```python
from build123d import *

# Parameters (mm, degrees)
F0_R     = 6
F1_DEPTH = 5
F2_DEPTH = 3
F3_W     = 34
F3_H     = 50
F4_DEPTH = 2
F5_R     = 1.155008
F5_R_2   = 1.094696
F5_R_3   = 1.161259
F5_R_4   = 0.979267
F6_DEPTH = 3.001


with BuildPart() as f1:
    # F0 (on Top) → F1 (new body)
    with BuildSketch(Plane.XY):
        with BuildLine():
            ThreePointArc((83.212636, 86.809125), (44.989895, 73.04652), (6.710183, 86.64986))
            ThreePointArc((6.710183, 86.64986), (-5.47746, 95.123225), (3.790625, 83.528434))
            ThreePointArc((3.790625, 83.528434), (15.91287, 45.057288), (3.24039, 6.763865))
            ThreePointArc((3.24039, 6.763865), (-5.358143, -5.247885), (6.829769, 3.099073))
            ThreePointArc((6.829769, 3.099073), (45.077454, 16.173317), (83.585051, 3.88567))
            ThreePointArc((83.585051, 3.88567), (94.910037, -5.66935), (87.070277, 6.904109))
            ThreePointArc((87.070277, 6.904109), (75.1752, 45.066281), (86.359609, 83.442748))
            ThreePointArc((86.359609, 83.442748), (95.478836, 95.121753), (83.212636, 86.809125))
        make_face()
        Circle(F0_R, mode=Mode.SUBTRACT)
        with Locations((90, 0)):
            Circle(F0_R, mode=Mode.SUBTRACT)
        with BuildLine():
            ThreePointArc((85.006812, 84.403744), (71.302344, 45), (85.006812, 5.596256))
            ThreePointArc((85.006812, 5.596256), (84.696699, 5.303301), (84.403744, 4.993188))
            ThreePointArc((84.403744, 4.993188), (45, 18.697656), (5.596256, 4.993188))
            ThreePointArc((5.596256, 4.993188), (5.303301, 5.303301), (4.993188, 5.596256))
            ThreePointArc((4.993188, 5.596256), (18.697656, 45), (4.993188, 84.403744))
            ThreePointArc((4.993188, 84.403744), (5.303301, 84.696699), (5.596256, 85.006812))
            ThreePointArc((5.596256, 85.006812), (45, 71.302344), (84.403744, 85.006812))
            ThreePointArc((84.403744, 85.006812), (84.696699, 84.696699), (85.006812, 84.403744))
        make_face(mode=Mode.SUBTRACT)
        with Locations((0, 90)):
            Circle(F0_R, mode=Mode.SUBTRACT)
        with Locations((90, 90)):
            Circle(F0_R, mode=Mode.SUBTRACT)
    extrude(amount=F1_DEPTH)

    # F0 (on Top) → F2 (join)
    with BuildSketch(Plane.XY):
        with BuildLine():
            ThreePointArc((84.403744, 4.993188), (84.696699, 5.303301), (85.006812, 5.596256))
            ThreePointArc((85.006812, 5.596256), (71.302344, 45), (85.006812, 84.403744))
            ThreePointArc((85.006812, 84.403744), (84.696699, 84.696699), (84.403744, 85.006812))
            ThreePointArc((84.403744, 85.006812), (45, 71.302344), (5.596256, 85.006812))
            ThreePointArc((5.596256, 85.006812), (5.303301, 84.696699), (4.993188, 84.403744))
            ThreePointArc((4.993188, 84.403744), (18.697656, 45), (4.993188, 5.596256))
            ThreePointArc((4.993188, 5.596256), (5.303301, 5.303301), (5.596256, 4.993188))
            ThreePointArc((5.596256, 4.993188), (45, 18.697656), (84.403744, 4.993188))
        make_face()
    extrude(amount=F2_DEPTH)

    # F3 (on face) → F4 (cut)
    with BuildSketch(Plane.XY.offset(3)):
        with Locations((45, 45)):
            Rectangle(F3_W, F3_H)
    extrude(amount=-F4_DEPTH, mode=Mode.SUBTRACT)

    # F5 (on face) → F6 (cut, through all)
    with BuildSketch(Plane.XY.offset(3)):
        with Locations((59.727397, 21.745855)):
            Circle(F5_R)
        with Locations((29.705523, 68.703085)):
            Circle(F5_R_2)
        with Locations((29.668592, 21.745855)):
            Circle(F5_R_3)
        with Locations((59.817981, 68.572104)):
            Circle(F5_R_4)
    extrude(amount=-F6_DEPTH, mode=Mode.SUBTRACT)


solid = f1.part
```
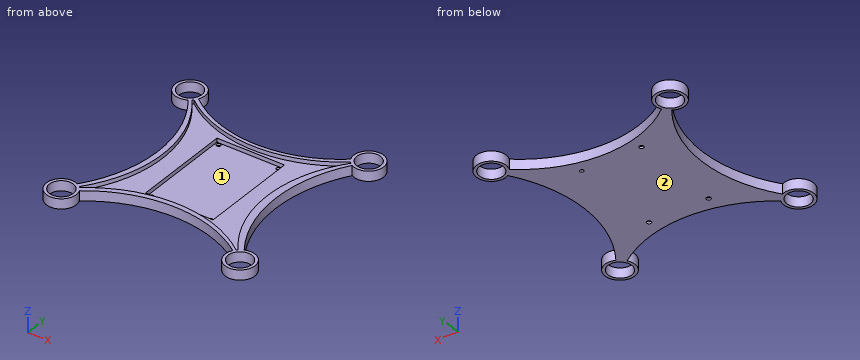
Read the model definition and answer for the solid it produces. Units are mm, in the model's axes. Face numbers are marked on the shaded views. Give positions to 0.01 mm unless a question says otherwise; leave off trailing zeros. Order: outer loops, then holes, each group sorted by start corner. A loop starts at its lowest first (then second) coordinate and runs counter-clockwise, first axis right, second up.
(1) Given pin 1 (3 mm diameter, centred on y = 50.5, z = 2.5, fed in from +X); pin 2 (0.6 mm diameter, centred on x = 43, z = 2.5, fed in from -Y); pin 3 (2 mm diameter, centred on x = 56, z = 1.5, fed in from +Y), each flat-ended and moving along its own axis, determine where each tip first touches the part or whether it passes through.
(2) For a pull along X with two mould halves and no side action, classify the marked faces 1 and 2 as released by +X, released by -X, zero draft, split by the parting line, or undercut.
(3) Find section A-A (y = 90). Give the vertices of the cut face in (x, z).
(4) Find section D-D (z = 3.75). Give the vertices of the cut face in (x, y).
(5) Straight lines are drawn through the part: L1, parallel to Y at x = 90, z = 2.3; L2, parallel to Y at x = 86.5, z = 3.4; L3, parallel to X at y = -3, z = 4.35. For each, find the intervals that lie inside material, in ascending order.
(6) Find section C-C (x = 13). Give the vertices of the cut face in (y, z), plus the area to 3 significant figures.
Result sheet:
1. pin 1: stops at x = 75.46
1. pin 2: stops at y = 16.11
1. pin 3: stops at y = 74.28
2. face 1: undercut
2. face 2: zero draft
3. outline: (-7.5, 0) - (-6, 0) - (-6, 5) - (-7.5, 5) - close; (6, 0) - (7.5, 0) - (7.5, 5) - (6, 5) - close; (82.5, 0) - (84, 0) - (84, 5) - (82.5, 5) - close; (96, 0) - (97.5, 0) - (97.5, 5) - (96, 5) - close
4. outline: (3.24, 6.76) arc R7.5 ccw (long way) to (6.83, 3.1) arc R64.42 cw to (83.59, 3.89) arc R7.5 ccw (long way) to (87.07, 6.9) arc R69.23 cw to (86.36, 83.44) arc R7.5 ccw (long way) to (83.21, 86.81) arc R60.31 cw to (6.71, 86.65) arc R7.5 ccw (long way) to (3.79, 83.53) arc R65.62 cw to start; hole circle Ø12 at (0, 0); hole circle Ø12 at (0, 90); hole (4.99, 5.6) arc R7.5 cw to (5.6, 4.99) arc R63.5 cw to (84.4, 4.99) arc R7.5 cw to (85.01, 5.6) arc R63.5 cw to (85.01, 84.4) arc R7.5 cw to (84.4, 85.01) arc R63.5 cw to (5.6, 85.01) arc R7.5 cw to (4.99, 84.4) arc R63.5 cw to start; hole circle Ø12 at (90, 0); hole circle Ø12 at (90, 90)
5. L1: y = -7.5 to -6, 6 to 7.5, 82.5 to 84, 96 to 97.5
5. L2: y = -6.63 to -4.87, 4.87 to 7.76, 83.37 to 85.13, 94.87 to 96.63
5. L3: x = -6.87 to -5.2, 5.2 to 6.87, 83.13 to 84.8, 95.2 to 96.87
6. outline: (7.24, 0) - (26.19, 0) - (26.19, 5) - (18.71, 5) - (18.71, 3) - (10.05, 3) - (10.05, 5) - (7.24, 5) - close; (64.87, 0) - (82.15, 0) - (82.15, 5) - (79.95, 5) - (79.95, 3) - (71.29, 3) - (71.29, 5) - (64.87, 5) - close
6. area: 147 mm2
